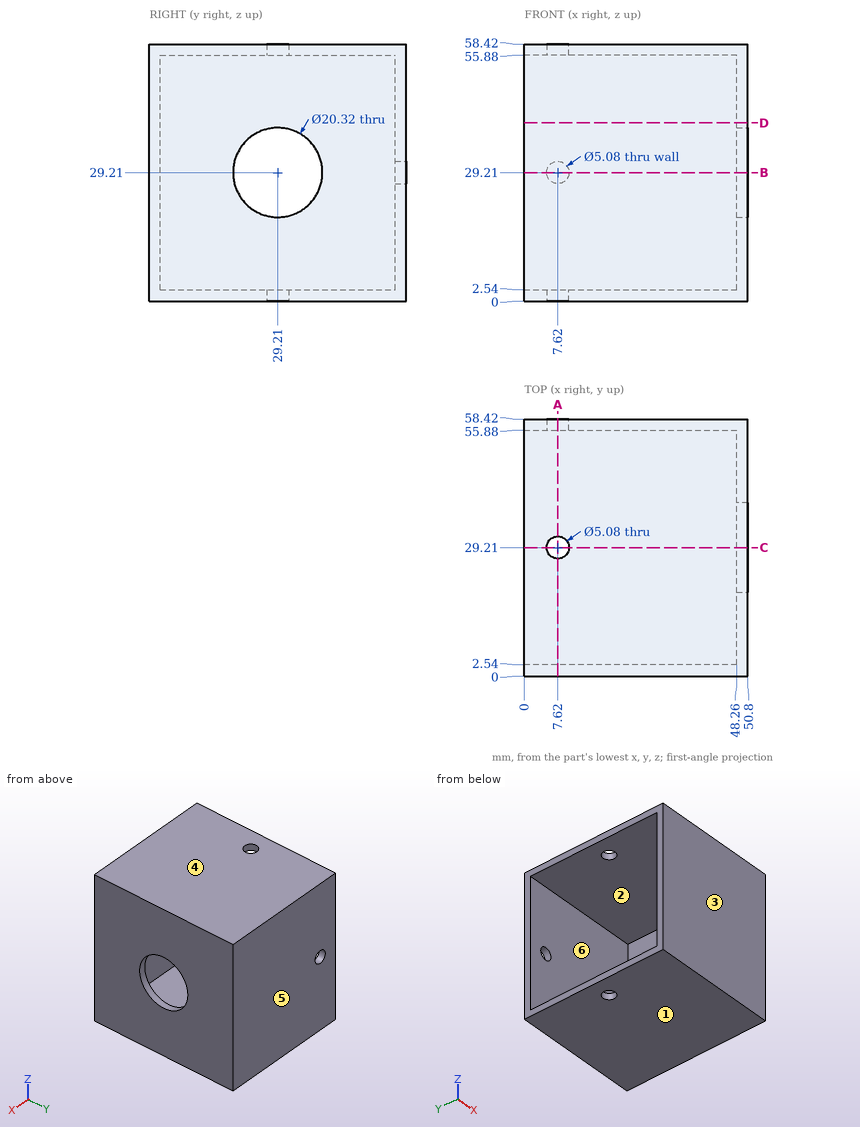
The drawing under review shows one solid part. Ordinate dimensions are in mm from its lowest x, y, z. A direction names the side the tool comes from. Give positions to 0.01 mm unless a question says otherwise; leave off trailing zeros. Write each loop counter-clockwise with the first axis right and the second up, starting at its lowest first coordinate (ties: lowest second). Pieces come first, ordered by that corner, then holes.
1. Add section C-C, the plane y = 29.21. Write out the cut boundary in (x, z).
2. Add section D-D, the plane z = 40.5. Write out the cut boundary in (x, y), plus the area to 3 significant figures.
3. Draft analysis for pull direction Z (two halves, no side actions). For the marked faces 1, 2, 3 and 4, state which applies: +Z half, -Z half, draft (parallel to the pull), parting line (faces both ways), or undercut.
4. Tool access review of the marked faces 5 and 6: name each direction out of +Z, -Z, +X, -X, +Y, -Y from which nothing blocks a thin tool from reaching the whole face with its end or side.
5. For P1, Ø1.5, axis at y = 10.5, z = 44.5, coming from the -X side, flat-tipped, find the tip position at first contact; note if it passes through.
6. Wall thickness on L1, parallel to X at y = 29, z = 1; L2, parallel to Z at x = 21.5, y = 14.5: over which ranges is each line inside the solid? List them lowest first.
7. Add section A-A, the plane x = 7.62. Write out the cut boundary in (y, z), plus the area to 3 significant figures.
8. Add section B-B, the plane z = 29.21. Write out the cut boundary in (x, y).
Worked answers:
1. outline: (0, 0) - (5.08, 0) - (5.08, 2.54) - (0, 2.54) - close; (0, 55.88) - (5.08, 55.88) - (5.08, 58.42) - (0, 58.42) - close; (10.16, 0) - (50.8, 0) - (50.8, 19.05) - (48.26, 19.05) - (48.26, 2.54) - (10.16, 2.54) - close; (10.16, 55.88) - (48.26, 55.88) - (48.26, 39.37) - (50.8, 39.37) - (50.8, 58.42) - (10.16, 58.42) - close
2. outline: (0, 0) - (50.8, 0) - (50.8, 58.42) - (0, 58.42) - (0, 55.88) - (48.26, 55.88) - (48.26, 2.54) - (0, 2.54) - close
2. area: 394 mm2
3. face 1: -Z half
3. face 2: undercut
3. face 3: draft
3. face 4: +Z half
4. face 5: +Z, -Z, +X, -X, +Y
4. face 6: -X
5. P1: stops at x = 48.26
6. L1: x = 0 to 5.09, 10.15 to 50.8
6. L2: z = 0 to 2.54, 55.88 to 58.42
7. outline: (0, 0) - (26.67, 0) - (26.67, 2.54) - (2.54, 2.54) - (2.54, 55.88) - (26.67, 55.88) - (26.67, 58.42) - (0, 58.42) - close; (31.75, 0) - (58.42, 0) - (58.42, 26.67) - (55.88, 26.67) - (55.88, 2.54) - (31.75, 2.54) - close; (31.75, 55.88) - (55.88, 55.88) - (55.88, 31.75) - (58.42, 31.75) - (58.42, 58.42) - (31.75, 58.42) - close
7. area: 529 mm2
8. outline: (0, 0) - (50.8, 0) - (50.8, 19.05) - (48.26, 19.05) - (48.26, 2.54) - (0, 2.54) - close; (0, 55.88) - (5.08, 55.88) - (5.08, 58.42) - (0, 58.42) - close; (10.16, 55.88) - (48.26, 55.88) - (48.26, 39.37) - (50.8, 39.37) - (50.8, 58.42) - (10.16, 58.42) - close
